Study the drawing (mm; zero at the part's minimum x, y, z) and answer. Round coordinates to 2 decimals unless told otherwise and drop trailing zeros. Order: outer loops, then holes, each group sorted by start corner. A loop starts at its lowest first (then second) coordinate and runs counter-clockwise, first axis right, second up. Notation, with made-up numbers: (-22, 23.25) - (35, 23.25) arc R32 ccw to (35, 52.25) - close; hole circle Ø11 at (25, 75.25). An arc over 180 degrees is marked (long way). Put each result on its own line as item: value. Start each with the question number.
Q1. For a pull along Z with two mould halves and no side action, classify the marked faces 1, 2 and 3 as pulls with the +Z half, pulls with the -Z half, needs draft (parallel to the pull), parting line crosses it, or undercut.
Q2. Section A-A on x = 10 is taken. Give the vertices of the cut face in (y, z).
Q3. Each of these flat-tipped pins is pushed along its axis until it touches: pin 1 Ø2 at (x, y) = (17, 10) entering from -Z; pin 2 Ø5 at (y, z) = (3.5, 4) entering from +X; pin 3 Ø1.5 at (y, z) = (16, 12) entering from -X. Where does it stop, or does it pass through?
Q4. Find the intervals of material crossed by line 1 along X through (y, z) = (11.75, 10); line 2 along Y through (x, z) = (8, 18); line 3 along Z through (x, y) = (11.5, 1.5), in increasing order. Write a range as from..to.
Q5. Section B-B on z = 10 is taken. Give the vertices of the cut face in (x, y).
Q6. Section C-C on y = 15.5 is taken. Give the vertices of the cut face in (x, z), then the cut area to 3 significant figures.
Q7. Section D-D on x = 16 is taken. Give the vertices of the cut face in (y, z), then the cut area to 3 significant figures.
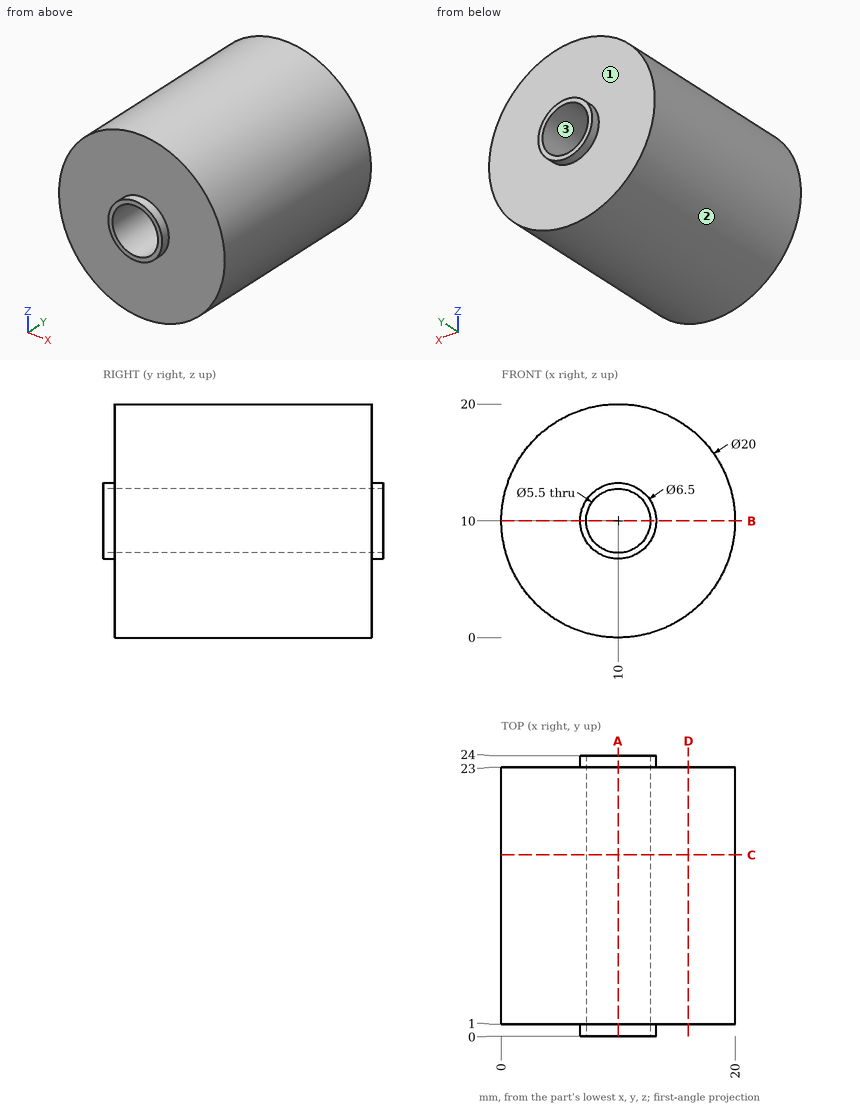
Findings:
1. face 1: needs draft
1. face 2: parting line crosses it
1. face 3: undercut
2. outline: (0, 6.75) - (1, 6.75) - (1, 0) - (23, 0) - (23, 6.75) - (24, 6.75) - (24, 7.25) - (0, 7.25) - close; (0, 12.75) - (24, 12.75) - (24, 13.25) - (23, 13.25) - (23, 20) - (1, 20) - (1, 13.25) - (0, 13.25) - close
3. pin 1: z = 2
3. pin 2: x = 19.37
3. pin 3: x = 0.08
4. line 1: 0..7.25, 12.75..20
4. line 2: 1..23
4. line 3: 0.11..7.7, 12.3..19.89
5. outline: (0, 1) - (6.75, 1) - (6.75, 0) - (7.25, 0) - (7.25, 24) - (6.75, 24) - (6.75, 23) - (0, 23) - close; (12.75, 0) - (13.25, 0) - (13.25, 1) - (20, 1) - (20, 23) - (13.25, 23) - (13.25, 24) - (12.75, 24) - close
6. outline: circle Ø20 at (10, 10); hole circle Ø5.5 at (10, 10)
6. area: 290 mm2
7. outline: (1, 2) - (23, 2) - (23, 18) - (1, 18) - close
7. area: 352 mm2
